from build123d import *

# Parameters (mm, degrees)
F1_DEPTH = 4
F2_R     = 2.4
F3_DEPTH = 55
F4_R     = 1.5
F5_DEPTH = 40


with BuildPart() as f1:
    # F0 (on Top) → F1 (new body)
    with BuildSketch(Plane.XY):
        Polygon((-0.031572, -5.773503), (4.984214, -2.914093), (5.015786, 2.859409), (0.031572, 5.773503), (-4.984214, 2.914093), (-5.015786, -2.859409), align=None)
    extrude(amount=F1_DEPTH)

    # F2 (on face) → F3 (join)
    with BuildSketch(Plane.XY):
        Circle(F2_R)
    extrude(amount=F3_DEPTH)

    # F4 (on Top) → F5 (cut)
    with BuildSketch(Plane.XY):
        Circle(F4_R)
    extrude(amount=F5_DEPTH, mode=Mode.SUBTRACT)


solid = f1.part
Part model, mm, in its own coordinate system. A direction names the side the tool comes from. Coordinates: 2 decimals unless noted, no trailing zeros. Loops run counter-clockwise (first coordinate to the right, second up) from the corner with the lowest first, then second, coordinate; pieces in that order, holes last. Notation, with made-up numbers: (-12, 68) - (45, 68) arc R24 ccw to (45, 100) - close; hole circle Ø3 at (58, 82). An arc over 180 degrees is marked (long way). Write each question's results on one line, items separated by ' | '. Start each with the question number.
Q1. Slice it at D-D on z = 48. Give the cut face in (x, y).
Q2. Two-plate mould, pull along Y, no slides. Class faces 1 (the flat face through (-2.559, -4.296, 1.972)), 2 (the cylindrical face through (-1.5, 0.07, 19.72)), 3 (the flat face through (-1.2, -1.2, 0)): +Y half, -Y half, draft (parallel to the pull), parting line (faces both ways), or undercut.
Q3. Slice it at B-B on z = 35. Give the cut face in (x, y), and give its area (3 significant figures).
Q4. Probe line 1 along Z through (x, y) = (0.75, 4.5); line 2 along X through (y, z) = (-0.5, 37); line 3 along Y through (x, z) = (0, 16). List the from-to ranges inside material, lowest first.
Q5. Which spindle directions (+Z, -Z, +X, -X, +Y, -Y) get a long thin tool onto all of the face, cutting with end or side? Do faces 4 (the flat face through (2.441, -4.364, 1.972)), 5 (the cylindrical face through (1.29, 2.024, 29.143)), 6 (the flat face through (0, 0, 40)). Say none if no direction does.
Q6. Drop flat-ended pins along their axis: pin 1 Ø1.5 at (x, y) = (3.5, -4) entering from +Z; pin 2 Ø4 at (x, z) = (-0.5, 29.5) entering from -Y; pin 3 Ø3 at (y, z) = (-4.5, 39) entering from +X; pin 4 Ø6 at (x, z) = (2, 45.5) entering from +Y. Give the stop position or say it passes through.
Q7. Slice it at C-C on x = -3.5. Give the cut face in (y, z), and give its area (3 significant figures).
Q8. Slice it at A-A on y = 0. Give the cut face in (x, z), and give its area (3 significant figures).
Answer:
1) outline: circle Ø4.8 at (0, 0)
2) face 1: -Y half | face 2: undercut | face 3: draft
3) outline: circle Ø4.8 at (0, 0); hole circle Ø3 at (0, 0) | area: 11.0 mm2
4) line 1: z = 0 to 4 | line 2: x = -2.35 to -1.41, 1.41 to 2.35 | line 3: y = -2.4 to -1.5, 1.5 to 2.4
5) face 4: +Z, -Z, +X, -Y | face 5: +Z | face 6: -Z
6) pin 1: stops at z = 4 | pin 2: stops at y = -2.4 | pin 3: passes through | pin 4: stops at y = 2.4
7) outline: (-3.75, 0) - (3.76, 0) - (3.76, 4) - (-3.75, 4) - close | area: 30.0 mm2
8) outline: (-5, 0) - (-1.5, 0) - (-1.5, 40) - (1.5, 40) - (1.5, 0) - (5, 0) - (5, 4) - (2.4, 4) - (2.4, 55) - (-2.4, 55) - (-2.4, 4) - (-5, 4) - close | area: 165 mm2
